from build123d import *
from OCP.BRepFilletAPI import BRepFilletAPI_MakeChamfer

# Parameters (mm, degrees)
SKETCH1_R           = 3.75
BOSS_EXTRUDE1_DEPTH = 6.5
CHAMFER1_SIZE       = 1
CHAMFER1_SIZE2      = 0.577350269


with BuildPart() as part:
    # Sketch1 → Boss-Extrude1 (new body)
    with BuildSketch(Plane(origin=(0, 0, 0), x_dir=(1, 0, 0), z_dir=(0, 1, 0))):
        with BuildLine():
            Line((-6, 0), (-6, 65))
            Line((-6, 65), (6, 65))
            Line((6, 65), (6, 0))
            ThreePointArc((6, 0), (0, -6), (-6, 0))
        make_face()
        with Locations(Location((0, 0, 0), (0, 0, 90))):
            Circle(SKETCH1_R, mode=Mode.SUBTRACT)
    extrude(amount=BOSS_EXTRUDE1_DEPTH)

    # Chamfer1: one chamfer whose edges measure the first distance from different faces: ONE call of the kernel's chamfer builder (chamfer() names one face for all edges)
    chamfer1_edges_1 = [part.edges().sort_by_distance(p)[0] for p in [
        (0, 6.5, -65),
    ]]
    chamfer1_side_1 = [part.faces().sort_by_distance(p)[0] for p in [
        (0, 6.5, -31.810895579),
    ]]
    chamfer1_edges_2 = [part.edges().sort_by_distance(p)[0] for p in [
        (0, 0, -65),
    ]]
    chamfer1_side_2 = [part.faces().sort_by_distance(p)[0] for p in [
        (0, 0, -31.810895579),
    ]]
    chamfer1_edges_3 = [part.edges().sort_by_distance(p)[0] for p in [
        (-6, 3.25, -65),
    ]]
    chamfer1_side_3 = [part.faces().sort_by_distance(p)[0] for p in [
        (-6, 3.25, -32.5),
    ]]
    chamfer1_edges_4 = [part.edges().sort_by_distance(p)[0] for p in [
        (6, 3.25, -65),
    ]]
    chamfer1_side_4 = [part.faces().sort_by_distance(p)[0] for p in [
        (6, 3.25, -32.5),
    ]]
    chamfer1 = BRepFilletAPI_MakeChamfer(part.part.solid().wrapped)
    for e in chamfer1_edges_1:
        chamfer1.Add(CHAMFER1_SIZE, CHAMFER1_SIZE2, e.wrapped, chamfer1_side_1[0].wrapped)  # the first distance lies on this face
    for e in chamfer1_edges_2:
        chamfer1.Add(CHAMFER1_SIZE, CHAMFER1_SIZE2, e.wrapped, chamfer1_side_2[0].wrapped)  # the first distance lies on this face
    for e in chamfer1_edges_3:
        chamfer1.Add(CHAMFER1_SIZE, CHAMFER1_SIZE2, e.wrapped, chamfer1_side_3[0].wrapped)  # the first distance lies on this face
    for e in chamfer1_edges_4:
        chamfer1.Add(CHAMFER1_SIZE, CHAMFER1_SIZE2, e.wrapped, chamfer1_side_4[0].wrapped)  # the first distance lies on this face
    add(Compound.cast(chamfer1.Shape()), mode=Mode.REPLACE)


solid = part.part
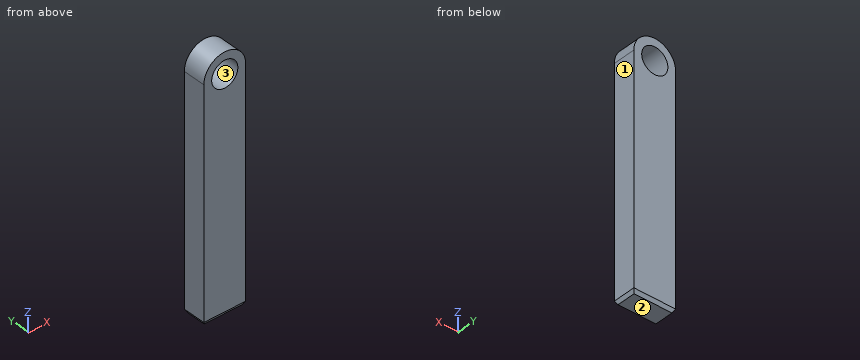
Here's how the part is built. I have some questions about the finished solid (model axes, mm). Face numbers are marked on the shaded views. Round coordinates to 2 decimals unless told otherwise and drop trailing zeros. Write each loop counter-clockwise with the first axis right and the second up, starting at its lowest first coordinate (ties: lowest second). Pieces come first, ordered by that corner, then holes. Notation, with made-up numbers: (-14, -17.75) -> (28, -17.75) arc R19 cw to (28, -2.75) -> close; hole circle Ø6 at (38.25, 34). An arc over 180 degrees is marked (long way). One line per item, written item: value.
1) We'd pull the mould along Z, two halves only. Please class the marked faces 1, 2 and 3: released by +Z, released by -Z, zero draft, split by the parting line, or undercut.
Filled sheet:
face 1: zero draft
face 2: released by -Z
face 3: undercut
2) Suppose I cut it at D-D on x = -4.5. List the corners of the cut face in (y, z) for me, plus the area to 3 significant figures.
Filled sheet:
outline: (0, -64) -> (0.58, -65) -> (5.92, -65) -> (6.5, -64) -> (6.5, 3.97) -> (0, 3.97) -> close
area: 448 mm2
3) Suppose I cut it at C-C on z = -2. List the corners of the cut face in (x, y) for me.
Filled sheet:
outline: (-6, 0) -> (-3.17, 0) -> (-3.17, 6.5) -> (-6, 6.5) -> close; (3.17, 0) -> (6, 0) -> (6, 6.5) -> (3.17, 6.5) -> close
4) Suppose I cut it at A-A on x = 0. List the corners of the cut face in (y, z) for me, plus the area to 3 significant figures.
Filled sheet:
outline: (0, -64) -> (0.58, -65) -> (5.92, -65) -> (6.5, -64) -> (6.5, -3.75) -> (0, -3.75) -> close; (0, 3.75) -> (6.5, 3.75) -> (6.5, 6) -> (0, 6) -> close
area: 412 mm2
5) Suppose I cut it at B-B on y = 4.5. List the corners of the cut face in (x, z) for me, plus the area to 3 significant figures.
Filled sheet:
outline: (-6, -64) -> (-5.42, -65) -> (5.42, -65) -> (6, -64) -> (6, 0) arc R6 ccw to (-6, 0) -> close; hole circle Ø7.5 at (0, 0)
area: 792 mm2
6) If I drill on line 1 (X direction, y = 4, z = 0); line 2 (Z direction, x = -2.5, y = 5); line 3 (Z direction, x = -1, y = 5.25), over which ranges is the centre line in solid material (lowest first)? Write a range as [from, to].
Filled sheet:
line 1: x = [-6, -3.75], [3.75, 6]
line 2: z = [-65, -2.8], [2.8, 5.45]
line 3: z = [-65, -3.61], [3.61, 5.92]
